The listing builds one solid part. Answer for the finished solid, in the listing's coordinates (mm). A direction names the side the tool comes from. Coordinates: 2 decimals unless noted, no trailing zeros. Write each loop counter-clockwise with the first axis right and the second up, starting at its lowest first coordinate (ties: lowest second). Pieces come first, ordered by that corner, then holes.
from build123d import *

# Parameters (mm, degrees)
SKETCH1_W           = 40.386
SKETCH1_H           = 40.894
BOSS_EXTRUDE1_DEPTH = 9.906
SKETCH2_W           = 56.388
SKETCH2_H           = 3.175
BOSS_EXTRUDE2_DEPTH = 19.812
SKETCH3_R           = 2.159
CUT_EXTRUDE1_DEPTH  = 19.812
SKETCH4_R           = 2.032
BOSS_EXTRUDE3_DEPTH = 6.35


with BuildPart() as part:
    # Sketch1 → Boss-Extrude1 (new, symmetric)
    with BuildSketch(Plane(origin=(0, 0, 0), x_dir=(0, 0, -1), z_dir=(1, 0, 0))):
        Rectangle(SKETCH1_W, SKETCH1_H)
    extrude(amount=BOSS_EXTRUDE1_DEPTH, both=True)

    # Sketch2 → Boss-Extrude2 (add, through all)
    with BuildSketch(Plane(origin=(9.906, 0, 0), x_dir=(0, 0, -1), z_dir=(1, 0, 0))):
        with Locations((0, 5.9055)):
            Rectangle(SKETCH2_W, SKETCH2_H)
    extrude(amount=-BOSS_EXTRUDE2_DEPTH)

    # Sketch3 → Cut-Extrude1 (cut)
    with BuildSketch(Plane(origin=(0, 7.493, 0), x_dir=(1, 0, 0), z_dir=(0, 1, 0))):
        with Locations(Location((-4.953, 23.876, 0), (0, 0, 270))):
            Circle(SKETCH3_R)
        with Locations(Location((4.953, 23.876, 0), (0, 0, 270))):
            Circle(SKETCH3_R)
        with Locations(Location((4.953, -23.876, 0), (0, 0, 270))):
            Circle(SKETCH3_R)
        with Locations(Location((-4.953, -23.876, 0), (0, 0, 270))):
            Circle(SKETCH3_R)
    extrude(amount=-CUT_EXTRUDE1_DEPTH, mode=Mode.SUBTRACT)

    # Sketch4 → Boss-Extrude3 (add)
    with BuildSketch(Plane(origin=(0, 20.447, 0), x_dir=(1, 0, 0), z_dir=(0, 1, 0))):
        with Locations(Location((0, -11.303, 0), (0, 0, 90))):
            Circle(SKETCH4_R)
    extrude(amount=BOSS_EXTRUDE3_DEPTH)


solid = part.part
Q1. The part is cut by section A-A, the plane x = 0. Write down the section's boundary in (y, z) (3 decimals), then the cut area to 3 significant figures.
Answers below:
outline: (-20.447, -20.193) - (4.318, -20.193) - (4.318, -28.194) - (7.493, -28.194) - (7.493, -20.193) - (20.447, -20.193) - (20.447, 9.271) - (26.797, 9.271) - (26.797, 13.335) - (20.447, 13.335) - (20.447, 20.193) - (7.493, 20.193) - (7.493, 28.194) - (4.318, 28.194) - (4.318, 20.193) - (-20.447, 20.193) - close
area: 1,730 mm2
Q2. Determine the mould class of faces 1 (the face through (0, -20.447, 0)), 2 (the face through (-0.61, 23.578, 9.365)), 3 (the face through (5.05, 5.93, 21.72)) for opening direction X: released by +X, released by -X, zero draft, split by the parting line, or undercut.
Answers below:
face 1: zero draft
face 2: split by the parting line
face 3: undercut
Q3. The part is cut by section D-D, the plane x = 4. Write down the section's boundary in (y, z).
Answers below:
outline: (-20.45, -20.19) - (4.32, -20.19) - (4.32, -21.94) - (7.49, -21.94) - (7.49, -20.19) - (20.45, -20.19) - (20.45, 20.19) - (7.49, 20.19) - (7.49, 21.94) - (4.32, 21.94) - (4.32, 20.19) - (-20.45, 20.19) - close; (4.32, -28.19) - (7.49, -28.19) - (7.49, -25.81) - (4.32, -25.81) - close; (4.32, 25.81) - (7.49, 25.81) - (7.49, 28.19) - (4.32, 28.19) - close
Q4. The part is cut by section B-B, the plane y = 6.5. Write down the section's boundary in (x, z) (3 decimals), then the cut area to 3 significant figures.
Answers below:
outline: (-9.906, -28.194) - (9.906, -28.194) - (9.906, 28.194) - (-9.906, 28.194) - close; hole circle Ø4.318 at (-4.953, -23.876); hole circle Ø4.318 at (-4.953, 23.876); hole circle Ø4.318 at (4.953, -23.876); hole circle Ø4.318 at (4.953, 23.876)
area: 1,060 mm2
Q5. Given pin 1 (6 mm diameter, centred on x = -4, y = -1, fed in from +Z); pin 2 (8 mm diameter, centred on x = -7.5, z = 5, fed in from +Y); pin 3 (3 mm diameter, centred on x = -5.5, y = -7.5, fed in from -Z); pin 4 (3.5 mm diameter, centred on x = 4.953, z = 23.876, fed in from +Y), each flat-ended and moving along its own axis, determine where each tip first touches the part or whether it passes through.
Answers below:
pin 1: stops at z = 20.19
pin 2: stops at y = 20.45
pin 3: stops at z = -20.19
pin 4: passes through
Q6. Which of the six approach directions +Z, -Z, +X, -X, +Y, -Y give full straight-line access (tool end or side, diameter ignored) to faces 4 (the face through (0, 7.493, 24)), 5 (the face through (0, -8, 20.193)), 6 (the face through (0, 4.318, -24)), 7 (the face through (0, 14, -20.193))?
Answers below:
face 4: +Z, +X, -X, +Y
face 5: +Z, +X, -X, -Y
face 6: -Z, +X, -X, -Y
face 7: -Z, +X, -X, +Y
Q7. Find the intervals of material crossed by probe 1 along Y at (x, z) = (-2, 22.5); probe 2 along Z at (x, y) = (5.25, -1); probe 3 along Y at (x, z) = (-2.5, -7), in increasing order.
Answers below:
probe 1: y = 4.32 to 7.49
probe 2: z = -20.19 to 20.19
probe 3: y = -20.45 to 20.45
Q8. The part is cut by section C-C, the plane z = -16.5. Write down the section's boundary in (x, y), then the cut area to 3 significant figures.
Answers below:
outline: (-9.91, -20.45) - (9.91, -20.45) - (9.91, 20.45) - (-9.91, 20.45) - close
area: 810 mm2
